CAD build for the part. Positions are in the model's coordinates, mm. A direction names the side the tool comes from. Give positions to 0.01 mm unless a question says otherwise; leave off trailing zeros. Loops run counter-clockwise (first coordinate to the right, second up) from the corner with the lowest first, then second, coordinate; pieces in that order, holes last.
```python
from build123d import *

# Parameters (mm, degrees)
SKETCH_R     = 20.5
PAD_DEPTH    = 2
SKETCH001_R  = 19.5
PAD001_DEPTH = 2
SKETCH002_W  = 34
SKETCH002_H  = 5.8
PAD002_DEPTH = 4
SKETCH003_W  = 30.1
SKETCH003_H  = 1.8
POCKET_DEPTH = 3


with BuildPart() as part:
    # Sketch → Pad (new body)
    with BuildSketch(Plane.XY):
        Circle(SKETCH_R)
    extrude(amount=PAD_DEPTH)

    # Sketch001 (on Face3 of Pad) → Pad001 (join)
    with BuildSketch(Plane.XY.offset(2)):
        Circle(SKETCH001_R)
    extrude(amount=PAD001_DEPTH)

    # Sketch002 (on Face5 of Pad001) → Pad002 (join)
    with BuildSketch(Plane.XY.offset(4)):
        Rectangle(SKETCH002_W, SKETCH002_H)
    extrude(amount=PAD002_DEPTH)

    # Sketch003 (on Face10 of Pad002) → Pocket (cut)
    with BuildSketch(Plane.XY.offset(8)):
        Rectangle(SKETCH003_W, SKETCH003_H)
    extrude(amount=-POCKET_DEPTH, mode=Mode.SUBTRACT)


solid = part.part
```
1. Pull direction Y, two halves, no side cores. Call faces 1 (the face through (0, 0, 5)), 2 (the face through (11, -17, 2)), 3 (the face through (0, -2.9, 6)), 4 (the face through (0, 0.9, 7)): released by +Y, released by -Y, zero draft, split by the parting line, or undercut.
Responses:
face 1: undercut
face 2: zero draft
face 3: released by -Y
face 4: undercut
2. Saw through at C-C, the plane x = 0. List the corners of the cut face in (y, z).
Responses:
outline: (-20.5, 0) - (20.5, 0) - (20.5, 2) - (19.5, 2) - (19.5, 4) - (2.9, 4) - (2.9, 8) - (0.9, 8) - (0.9, 5) - (-0.9, 5) - (-0.9, 8) - (-2.9, 8) - (-2.9, 4) - (-19.5, 4) - (-19.5, 2) - (-20.5, 2) - close
3. Saw through at A-A, the plane z = 7. List the corners of the cut face in (x, y).
Responses:
outline: (-17, -2.9) - (17, -2.9) - (17, 2.9) - (-17, 2.9) - close; hole (-15.05, -0.9) - (15.05, -0.9) - (15.05, 0.9) - (-15.05, 0.9) - close
4. Drop flat-ended pins along their axis: pin 1 (0.9 mm diameter, centred on x = -7, z = 6.5, fed in from +Y); pin 2 (2 mm diameter, centred on y = 0, z = 6.5, fed in from +X); pin 3 (1 mm diameter, centred on x = 13, z = 7, fed in from -Y). Give the stop position or say it passes through.
Responses:
pin 1: stops at y = 2.9
pin 2: stops at x = 17
pin 3: stops at y = -2.9
5. Tool access for faces 5 (the face through (17, 0, 6)), 6 (the face through (-17, 0, 6)), 7 (the face through (-2.539, 19.334, 2.986)): list every direction of +Z, -Z, +X, -X, +Y, -Y with a clear straight run to the whole face (end or side of a thin tool).
Responses:
face 5: +Z, +X, +Y, -Y
face 6: +Z, -X, +Y, -Y
face 7: +Z
6. Probe line 1 along Y through (x, z) = (13, 5.25); line 2 along Z through (x, y) = (3, -4); line 3 along X through (y, z) = (1, 6.5). List the from-to ranges inside material, lowest first.
Responses:
line 1: y = -2.9 to -0.9, 0.9 to 2.9
line 2: z = 0 to 4
line 3: x = -17 to 17
7. Saw through at D-D, the plane z = 4.5. List the corners of the cut face in (x, y), and give its area (3 significant figures).
Responses:
outline: (-17, -2.9) - (17, -2.9) - (17, 2.9) - (-17, 2.9) - close
area: 197 mm2
8. Saw through at B-B, the plane y = 0. List the corners of the cut face in (x, z).
Responses:
outline: (-20.5, 0) - (20.5, 0) - (20.5, 2) - (19.5, 2) - (19.5, 4) - (17, 4) - (17, 8) - (15.05, 8) - (15.05, 5) - (-15.05, 5) - (-15.05, 8) - (-17, 8) - (-17, 4) - (-19.5, 4) - (-19.5, 2) - (-20.5, 2) - close
